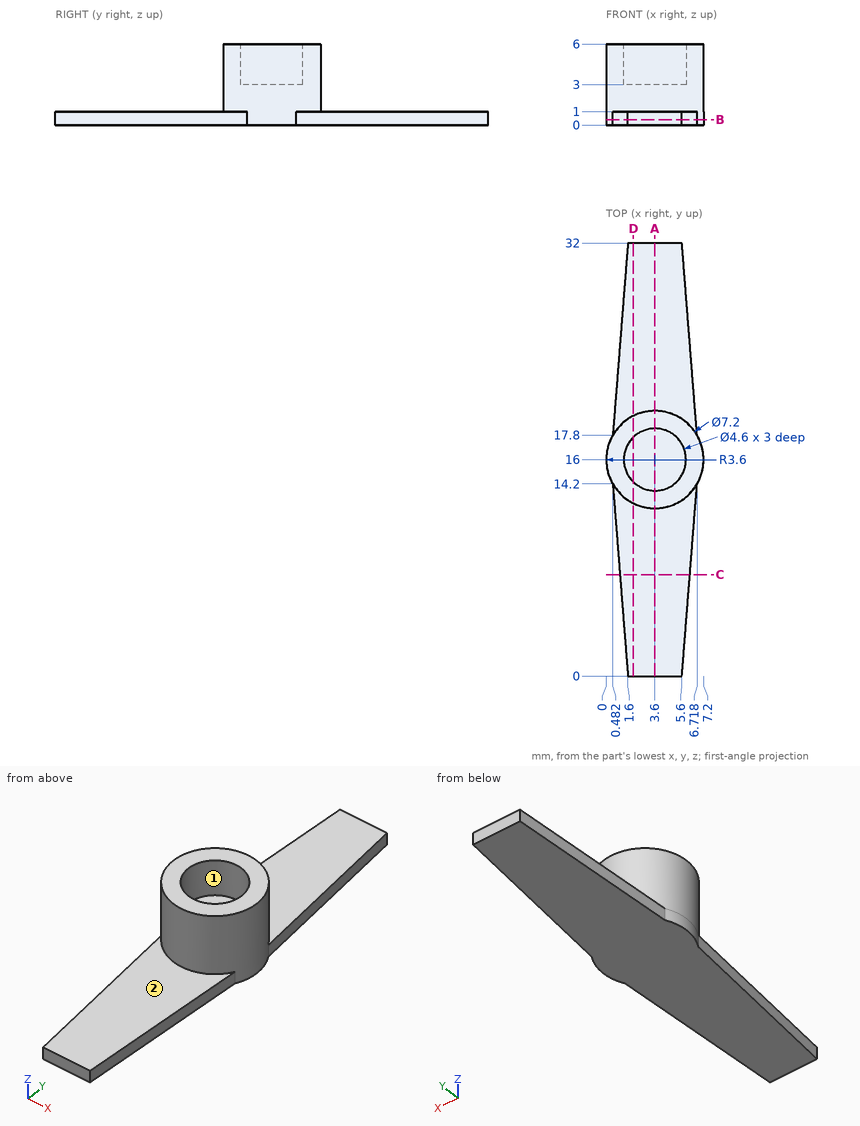
The figure shows three views and two pictorial views of one solid part (mm, origin at its lowest corner). Answer the questions. Coordinates: 2 decimals unless noted, no trailing zeros. Write each loop counter-clockwise with the first axis right and the second up, starting at its lowest first coordinate (ties: lowest second). Pieces come first, ordered by that corner, then holes. Notation, with made-up numbers: M -33,-27 L -5,-27 A22 ccw -5,-14 Z; hole C -36,27 d3. An arc over 180 degrees is marked long. Answer as CSV lines item,"result". Start each with the question number.
Item 1: Flat-ended cylindrical pins translate along their axes: P1, Ø1.5, axis at x = 4, y = 28.5, coming from the +Z side; P2, Ø1.4, axis at x = 2.5, y = 16, coming from the +Z side; P3, Ø1, axis at x = 3, z = 2, coming from the +Y side. Find the tip coordinate at first contact, or state that the pin passes through.
Item 2: Consider L1, parallel to Y at x = 3.6, z = 4.75; L2, parallel to Z at x = 4, y = 25; L3, parallel to Y at x = 2.5, z = 3.25. Determine where each line is inside the solid, lowest interval first.
Item 3: Section D-D on x = 2 is taken. Write down the section's boundary in (y, z) (1 decimal).
Item 4: Section C-C on y = 7.5 is taken. Write down the section's boundary in (x, z).
Item 5: Determine the mould class of the marked faces 1 and 2 for opening direction X: released by +X, released by -X, zero draft, split by the parting line, or undercut.
Item 6: Section A-A on x = 3.6 is taken. Write down the section's boundary in (y, z).
Item 7: Section B-B on z = 0.4 is taken. Write down the section's boundary in (x, y).
Checks:
1,P1,"stops at z = 1"
1,P2,"stops at z = 3"
1,P3,"stops at y = 19.6"
2,L1,"y = 12.4 to 13.7, 18.3 to 19.6"
2,L2,"z = 0 to 1"
2,L3,"y = 12.57 to 13.98, 18.02 to 19.43"
3,outline,"M 0,0 L 32,0 L 32,1 L 19.2,1 L 19.2,6 L 17.7,6 L 17.7,3 L 14.3,3 L 14.3,6 L 12.8,6 L 12.8,1 L 0,1 Z"
4,outline,"M 1.01,0 L 6.19,0 L 6.19,1 L 1.01,1 Z"
5,face 1,"undercut"
5,face 2,"zero draft"
6,outline,"M 0,0 L 32,0 L 32,1 L 19.6,1 L 19.6,6 L 18.3,6 L 18.3,3 L 13.7,3 L 13.7,6 L 12.4,6 L 12.4,1 L 0,1 Z"
7,outline,"M 0.48,14.2 L 1.6,0 L 5.6,0 L 6.72,14.2 A3.6 ccw 6.72,17.8 L 5.6,32 L 1.6,32 L 0.48,17.8 A3.6 ccw Z"
